For this review, use the dimensioned drawing (mm, ordinates from the lowest corner) and the shaded views. A direction names the side the tool comes from. Coordinates: 2 decimals unless noted, no trailing zeros. Write each loop counter-clockwise with the first axis right and the second up, starting at its lowest first coordinate (ties: lowest second). Pieces come first, ordered by that corner, then holes. Notation, with made-up numbers: M 86.25,-31 L 142.25,-31 A20 ccw 142.25,-14 Z; hole C -14.5,27.5 d10. An arc over 180 degrees is marked long. Return JSON: item names as keys, results as strings.
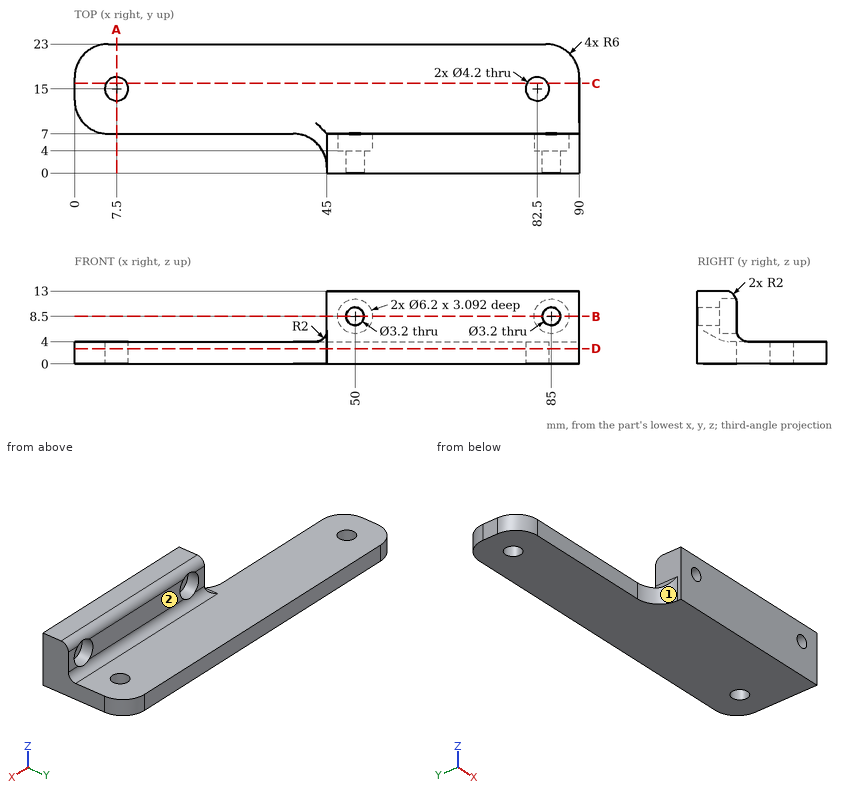
1. We need section D-D (z = 2.75). State the section outline as (x, y) points, plus the area to 3 significant figures.
Checks:
{"outline": "M 0,13 A6 ccw 6,7 L 39,7 A6 cw 45,1 L 45,0 L 90,0 L 90,17 A6 ccw 84,23 L 6,23 A6 ccw 0,17 Z; hole C 7.5,15 d4.2; hole C 82.5,15 d4.2", "area": "1,710 mm2"}
2. We need section C-C (y = 16). State the section outline as (x, z) points.
Checks:
{"outline": "M 0,0 L 5.65,0 L 5.65,4 L 0,4 Z; M 9.35,0 L 80.65,0 L 80.65,4 L 9.35,4 Z; M 84.35,0 L 90,0 L 90,4 L 84.35,4 Z"}
3. For the marked faces 1 and 2, list the 3-axis set-ups (+Z, -Z, +X, -X, +Y, -Y) from which the entire face can be reached by the end or side of a thin tool; tool diameter is ignored.
Checks:
{"face 1": "+Z, -Z, -X, -Y", "face 2": "+Z, +X, -X, +Y"}
4. We need section B-B (z = 8.5). State the section outline as (x, y) points, plus the area to 3 significant figures.
Checks:
{"outline": "M 45,0 L 48.4,0 L 48.4,4 L 46.9,4 L 46.9,7 L 45,7 Z; M 51.6,0 L 83.4,0 L 83.4,4 L 81.9,4 L 81.9,7 L 53.1,7 L 53.1,4 L 51.6,4 Z; M 86.6,0 L 90,0 L 90,7 L 88.1,7 L 88.1,4 L 86.6,4 Z", "area": "252 mm2"}
5. Clearance check with flat-ended pins moving along their axes: pin 1 Ø1 at (x, z) = (26, 6) entering from -Y; pin 2 Ø1.6 at (x, z) = (47, 9.5) entering from +Y; pin 3 Ø5 at (x, z) = (85, 8.5) entering from +Y; pin 4 Ø3.5 at (y, z) = (2, 5.5) entering from -X. State where each tip first meets the part, or that it passes through.
Checks:
{"pin 1": "through", "pin 2": "y = 7", "pin 3": "y = 4", "pin 4": "x = 44.45"}
6. We need section A-A (x = 7.5). State the section outline as (y, z) points, plus the area to 3 significant figures.
Checks:
{"outline": "M 7,0 L 12.9,0 L 12.9,4 L 7,4 Z; M 17.1,0 L 23,0 L 23,4 L 17.1,4 Z", "area": "47.2 mm2"}
7. Wall thickness on L1, parallel to X at y = 5.2, z = 8.5; L2, parallel to Z at x = 50, y = 1.85; L3, parallel to X at y = 5.5, z = 7.25: over which ranges is each line inside the solid? List them lowest first. Write a range as from..to.
Checks:
{"L1": "45..46.9, 53.1..81.9, 88.1..90", "L2": "0..6.9, 10.1..13", "L3": "45..47.16, 52.84..82.16, 87.84..90"}
